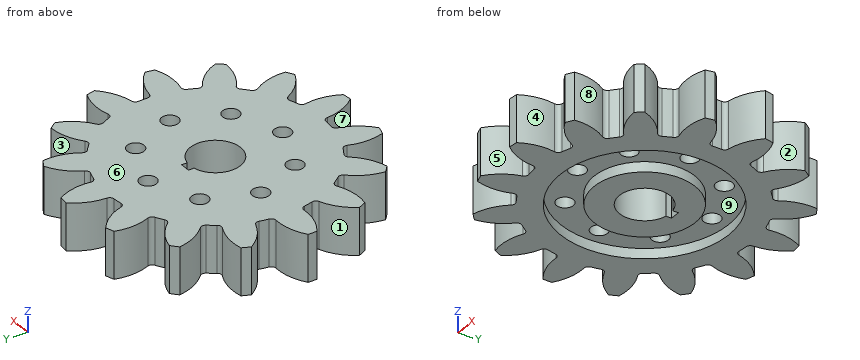
from build123d import *

# Parameters (mm, degrees)
SKETCH1_R           = 42.5
BOSS_EXTRUDE1_DEPTH = 14
CUT_EXTRUDE2_START  = -14
CUT_EXTRUDE2_DEPTH  = 14
CIRPATTERN1_COUNT   = 15
SKETCH3_R           = 25
CUT_EXTRUDE3_DEPTH  = 3
SKETCH4_R           = 7.5
CUT_EXTRUDE4_DEPTH  = 12
BOSS_EXTRUDE2_START = 3
SKETCH5_R           = 15
SKETCH5_R_2         = 7.5
BOSS_EXTRUDE2_DEPTH = 3
SKETCH6_R           = 2.5
CUT_EXTRUDE7_DEPTH  = 62.033988058
SKETCH7_W           = 3
SKETCH7_H           = 3
CUT_EXTRUDE8_DEPTH  = 62.645338009


with BuildPart() as part:
    # Sketch1 → Boss-Extrude1 (new body)
    with BuildSketch(Plane.XY):
        Circle(SKETCH1_R)
    extrude(amount=BOSS_EXTRUDE1_DEPTH)

    # Sketch2 → Cut-Extrude2 (cut)
    with BuildSketch(Plane.XY.offset(14).offset(CUT_EXTRUDE2_START)):
        with BuildLine():
            ThreePointArc((-2.144011648, 31.593985761), (-3.481811501, 31.474651879), (-4.813347736, 31.298696551))
            ThreePointArc((-4.813347736, 31.298696551), (-5.726736069, 31.495664334), (-6.276040886, 32.251533881))
            ThreePointArc((-6.276040886, 32.251533881), (-8.460316615, 36.991957647), (-12.087909655, 40.744722851))
            ThreePointArc((-12.087909655, 40.744722851), (-4.67296, 42.242318175), (2.890034901, 42.401623769))
            ThreePointArc((2.890034901, 42.401623769), (0.170397531, 37.946710693), (-0.924947108, 32.843486413))
            ThreePointArc((-0.924947108, 32.843486413), (-1.295759412, 31.98583101), (-2.144011648, 31.593985761))
        make_face()
    cut_extrude2 = extrude(amount=CUT_EXTRUDE2_DEPTH, mode=Mode.SUBTRACT)

    # CirPattern1: Cut-Extrude2 ×15 about axis
    cirpattern1_axis = Axis((0, 0, 0), (0, 0, 1))
    for i in range(1, CIRPATTERN1_COUNT):
        add(cut_extrude2.rotate(cirpattern1_axis, i * 360 / CIRPATTERN1_COUNT), mode=Mode.SUBTRACT)

    # Sketch3 → Cut-Extrude3 (cut)
    with BuildSketch(Plane(origin=(0, 0, 0), x_dir=(-1, 0, 0), z_dir=(0, 0, -1))):
        Circle(SKETCH3_R)
    extrude(amount=-CUT_EXTRUDE3_DEPTH, mode=Mode.SUBTRACT)

    # Sketch4 → Cut-Extrude4 (cut)
    with BuildSketch(Plane(origin=(0, 0, 3), x_dir=(-1, 0, 0), z_dir=(0, 0, -1))):
        Circle(SKETCH4_R)
    extrude(amount=-CUT_EXTRUDE4_DEPTH, mode=Mode.SUBTRACT)

    # Sketch5 → Boss-Extrude2 (add)
    with BuildSketch(Plane(origin=(0, 0, 3), x_dir=(-1, 0, 0), z_dir=(0, 0, -1)).offset(BOSS_EXTRUDE2_START)):
        Circle(SKETCH5_R)
        Circle(SKETCH5_R_2, mode=Mode.SUBTRACT)
    extrude(amount=-BOSS_EXTRUDE2_DEPTH)

    # Sketch6 → Cut-Extrude7 (cut, through all)
    with BuildSketch(Plane(origin=(0, 0, 3), x_dir=(-1, 0, 0), z_dir=(0, 0, -1))):
        with Locations((0, 20)):
            Circle(SKETCH6_R)
        with Locations((14.142135624, 14.142135624)):
            Circle(SKETCH6_R)
        with Locations((20, 0)):
            Circle(SKETCH6_R)
        with Locations((14.142135624, -14.142135624)):
            Circle(SKETCH6_R)
        with Locations((0, -20)):
            Circle(SKETCH6_R)
        with Locations((-14.142135624, -14.142135624)):
            Circle(SKETCH6_R)
        with Locations((-20, 0)):
            Circle(SKETCH6_R)
        with Locations((-14.142135624, 14.142135624)):
            Circle(SKETCH6_R)
    extrude(amount=-CUT_EXTRUDE7_DEPTH, mode=Mode.SUBTRACT)

    # Sketch7 → Cut-Extrude8 (cut, through all)
    with BuildSketch(Plane(origin=(0, 0, 0), x_dir=(-1, 0, 0), z_dir=(0, 0, -1))):
        with Locations((0, 7.5)):
            Rectangle(SKETCH7_W, SKETCH7_H)
    extrude(amount=-CUT_EXTRUDE8_DEPTH, mode=Mode.SUBTRACT)


solid = part.part
Read the model definition and answer for the solid it produces. Units are mm, in the model's axes. Face numbers are marked on the shaded views. A direction names the side the tool comes from. Coordinates: 2 decimals unless noted, no trailing zeros. Order: outer loops, then holes, each group sorted by start corner. A loop starts at its lowest first (then second) coordinate and runs counter-clockwise, first axis right, second up. Notation, with made-up numbers: M 21.5,-10 L 68.5,-10 A17 cw 68.5,13 Z; hole C 71.5,79 d3. An arc over 180 degrees is marked long. Put each result on its own line as item: value. Start each with the question number.
Item 1: Section D-D, the plane z = 1 is taken. Count the separate pieces of the cut face and the enclosed holes in it, plus the area to 3 significant figures.
Item 2: Given pin 1 Ø5 at (y, z) = (33.5, 6.5) entering from -X; pin 2 Ø3 at (x, y) = (-20, 0) entering from +Z; pin 3 Ø5 at (x, y) = (14, -11) entering from -Z; pin 4 Ø8 at (x, z) = (17.5, 8.5) entering from +Y, each flat-ended and moving along its own axis, determine where each tip first touches the part or whether it passes through.
Item 3: Section C-C, the plane y = -35 is taken. Determine the outline of the cut face in (x, z), plus the area to 3 significant figures.
Item 4: Section A-A, the plane y = 0 is taken. Determine the outline of the cut face in (x, z), plus the area to 3 significant figures.
Item 5: Section B-B, the plane x = -21 is taken. Determine the outline of the cut face in (y, z), plus the area to 3 significant figures.
Item 6: Consider probe 1 along X at (y, z) = (35, 13.25); probe 2 along Y at (x, z) = (20, 10); probe 3 along X at (y, z) = (12.5, 5.5). Determine where each line is inside the solid, lowest interval first. Write a range as [from, to].
Item 7: The mould has two halves that part along X. Classify the marked faces 6, 7, 8 and 9: +X half, -X half, draft (parallel to the pull), parting line (faces both ways), or undercut.
Item 8: For the marked faces 1, 2, 3, 4 and 5, determine the directions among +Z, -Z, +X, -X, +Y, -Y from which every point of the face is accessible in a straight line to the end or side of a thin tool.
Computed:
1. separate pieces: 2
1. enclosed holes: 2
1. area: 2,840 mm2
2. pin 1: stops at x = -29.07
2. pin 2: passes through
2. pin 3: stops at z = 3
2. pin 4: stops at y = 37.56
3. outline: M -14.9,0 L -6.88,0 L -6.88,14 L -14.9,14 Z; M -0.3,0 L 7.94,0 L 7.94,14 L -0.3,14 Z; M 16.6,0 L 22.64,0 L 22.64,14 L 16.6,14 Z
3. area: 312 mm2
4. outline: M -42.5,0 L -25,0 L -25,3 L -22.5,3 L -22.5,14 L -42.5,14 Z; M -17.5,3 L -15,3 L -15,0 L -7.5,0 L -7.5,14 L -17.5,14 Z; M 7.5,0 L 15,0 L 15,3 L 17.5,3 L 17.5,14 L 7.5,14 Z; M 22.5,3 L 25,3 L 25,0 L 31.67,0 L 31.67,14 L 22.5,14 Z
4. area: 658 mm2
5. outline: M -29.57,0 L -13.56,0 L -13.56,3 L -2.29,3 L -2.29,14 L -29.57,14 Z; M 2.29,3 L 13.56,3 L 13.56,0 L 29.08,0 L 29.08,14 L 2.29,14 Z
5. area: 689 mm2
6. probe 1: x = [-15.29, -7.3], [-0.68, 7.56], [16.02, 22.26]
6. probe 2: y = [-37.2, -25.94], [-24.67, -2.5], [2.5, 24.55], [26.61, 37.5]
6. probe 3: x = [-36.73, -16.03], [-12.26, 12.26], [16.03, 29.1]
7. face 6: draft
7. face 7: undercut
7. face 8: +X half
7. face 9: undercut
8. face 1: +Z, -Z, -X
8. face 2: +Z, -Z, +X
8. face 3: +Z, -Z, +Y
8. face 4: +Z, -Z
8. face 5: +Z, -Z, -Y
